Answer from the drawing. Dimensions are ordinates in mm from the lowest x, y and z of the part. A direction names the side the tool comes from. Round coordinates to 2 decimals unless told otherwise and drop trailing zeros. Write each loop counter-clockwise with the first axis right and the second up, starting at its lowest first coordinate (ties: lowest second). Pieces come first, ordered by that corner, then holes.
1. Find section A-A (y = 40.5). Write down the section's boundary in (x, z), and give its area (3 significant figures).
2. Straight lines are drawn through the part: probe 1 along Z at (x, y) = (21.5, 6.5); probe 2 along Z at (x, y) = (55.5, 38); probe 3 along X at (y, z) = (4, 28.5). For each, find the intervals that lie inside material, in ascending order.
3. Determine the mould class of the marked faces 1, 2, 3 and 4 for opening direction X: pulls with the +X half, pulls with the -X half, needs draft (parallel to the pull), parting line crosses it, or undercut.
4. Find section C-C (y = 17.5). Write down the section's boundary in (x, z), and give its area (3 significant figures).
5. Flat-ended cylindrical pins translate along their axes: pin 1 Ø3 at (y, z) = (2.5, 54) entering from +X; pin 2 Ø7 at (x, z) = (108, 10.5) entering from -Y; pin 3 Ø12 at (y, z) = (22, 50.5) entering from +X. Find the tip coordinate at first contact, or state that the pin passes through.
6. Find section B-B (x = 62). Write down the section's boundary in (y, z), and give its area (3 significant figures).
7. Find section D-D (z = 56). Write down the section's boundary in (x, y), and give its area (3 significant figures).
8. A tool of negligible diameter and unlimited length cuts with its end or side. For the marked faces 5, 6 and 7, from which of +Z, -Z, +X, -X, +Y, -Y can it reach the whole face along a straight path? Write none if from no direction.
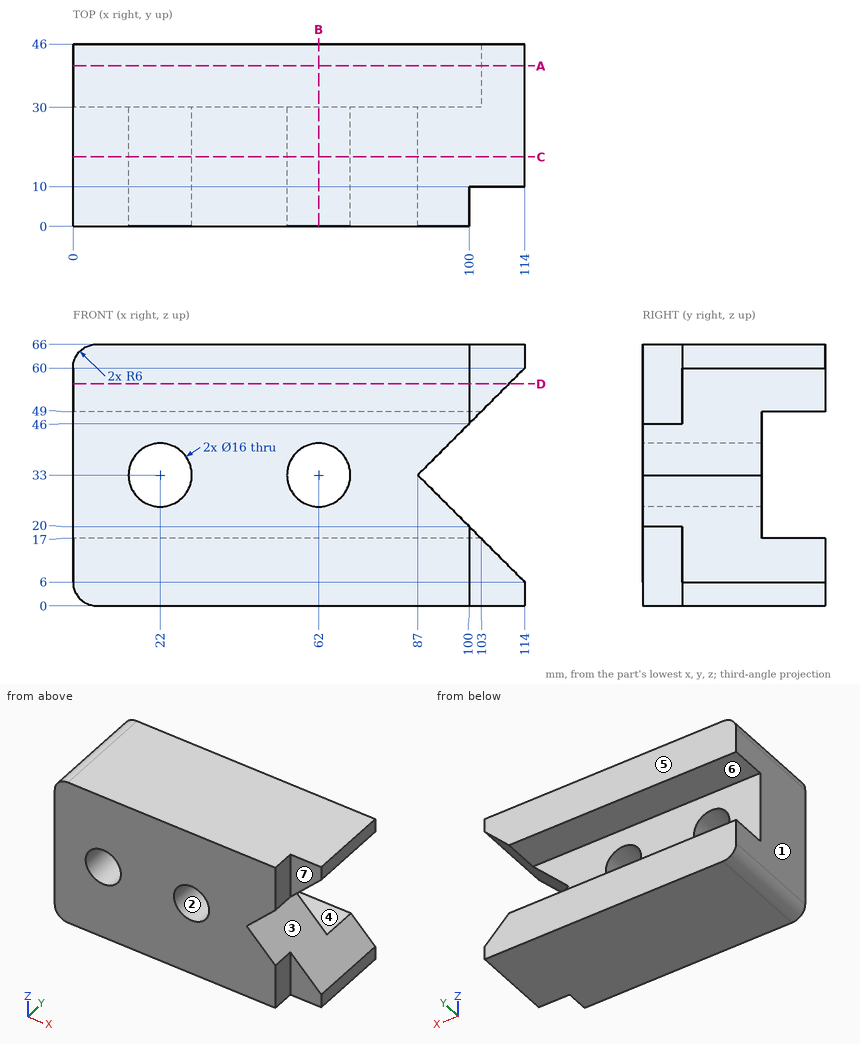
Worked answers:
1. outline: (0, 6) arc R6 ccw to (6, 0) - (114, 0) - (114, 6) - (103, 17) - (0, 17) - close; (0, 49) - (103, 49) - (114, 60) - (114, 66) - (6, 66) arc R6 ccw to (0, 60) - close
1. area: 3,740 mm2
2. probe 1: z = 0 to 25.02, 40.98 to 66
2. probe 2: z = 0 to 17, 49 to 66
2. probe 3: x = 0 to 15.39, 28.61 to 55.39, 68.61 to 91.5
3. face 1: pulls with the -X half
3. face 2: undercut
3. face 3: pulls with the +X half
3. face 4: needs draft
4. outline: (0, 6) arc R6 ccw to (6, 0) - (114, 0) - (114, 6) - (87, 33) - (114, 60) - (114, 66) - (6, 66) arc R6 ccw to (0, 60) - close; hole circle Ø16 at (22, 33); hole circle Ø16 at (62, 33)
4. area: 6,380 mm2
5. pin 1: stops at x = 100
5. pin 2: stops at y = 10
5. pin 3: stops at x = 110.5
6. outline: (0, 0) - (46, 0) - (46, 17) - (30, 17) - (30, 25) - (0, 25) - close; (0, 41) - (30, 41) - (30, 49) - (46, 49) - (46, 66) - (0, 66) - close
6. area: 2,040 mm2
7. outline: (0, 0) - (100, 0) - (100, 10) - (110, 10) - (110, 46) - (0, 46) - close
7. area: 4,960 mm2
8. face 5: +Z, -Z, +X, -X, +Y
8. face 6: +X, -X, +Y
8. face 7: +Z, -Z, +X, -Y
